Design review of the part built by this model. Coordinates are the model's own, in mm. A direction names the side the tool comes from. Give positions to 0.01 mm unless a question says otherwise; leave off trailing zeros. Write each loop counter-clockwise with the first axis right and the second up, starting at its lowest first coordinate (ties: lowest second). Pieces come first, ordered by that corner, then holes. Notation, with made-up numbers: (18.25, -28) - (43.25, -28) arc R13 ccw to (43.25, -14) - close; hole circle Ø2 at (60, -23). An arc over 180 degrees is marked (long way). Use a Markdown table: item, result. Add a question column.
```python
from build123d import *

# Parameters (mm, degrees)
ESQUISSE1_W                                       = 30
ESQUISSE1_H                                       = 30
BOSS_EXTRU_1_DEPTH                                = 38
ESQUISSE2_W                                       = 17.8
ESQUISSE2_H                                       = 4.4
ESQUISSE2_W_2                                     = 4.3
ESQUISSE2_H_2                                     = 17.8
ENL_V_MAT_EXTRU_1_DEPTH                           = 26
ESQUISSE3_W                                       = 26
ESQUISSE3_H                                       = 4.3
ENL_V_MAT_EXTRU_3_DEPTH                           = 31
ESQUISSE4_W                                       = 30
ESQUISSE4_H                                       = 3.85
BOSS_EXTRU_2_DEPTH                                = 12
FRAISAGE_POUR_VIS_T_TE_FRAIS_E_BOMB_E_D           = 5.09999996
FRAISAGE_POUR_VIS_T_TE_FRAIS_E_BOMB_E_CSINK_D     = 10.500000082
FRAISAGE_POUR_VIS_T_TE_FRAIS_E_BOMB_E_CSINK_ANGLE = 90


with BuildPart() as part:
    # Esquisse1 → Boss.-Extru.1 (new body)
    with BuildSketch(Plane(origin=(0, 0, 0), x_dir=(1, 0, 0), z_dir=(0, 1, 0))):
        with Locations((-20.886738322, -1.468531469)):
            Rectangle(ESQUISSE1_W, ESQUISSE1_H)
    extrude(amount=BOSS_EXTRU_1_DEPTH)

    # Esquisse2 → Enlèv. mat.-Extru.1 (cut)
    with BuildSketch(Plane.XZ):
        with Locations((-14.786738322, -7.431468531)):
            Rectangle(ESQUISSE2_W, ESQUISSE2_H)
        with Locations((-29.786738322, 7.568531469)):
            Rectangle(ESQUISSE2_W_2, ESQUISSE2_H_2)
        with Locations((-14.786738322, 7.568531469)):
            Rectangle(ESQUISSE2_W, ESQUISSE2_H_2)
    extrude(amount=-ENL_V_MAT_EXTRU_1_DEPTH, mode=Mode.SUBTRACT)

    # Esquisse3 → Enlèv. mat.-Extru.3 (cut, through all)
    with BuildSketch(Plane.XY.offset(16.468531469)):
        with Locations((-18.886738322, 32)):
            Rectangle(ESQUISSE3_W, ESQUISSE3_H)
    extrude(amount=-ENL_V_MAT_EXTRU_3_DEPTH, mode=Mode.SUBTRACT)

    # Esquisse4 → Boss.-Extru.2 (add)
    with BuildSketch(Plane(origin=(0, 0, -13.531468531), x_dir=(-1, 0, 0), z_dir=(0, 0, -1))):
        with Locations((20.886738322, 36.075)):
            Rectangle(ESQUISSE4_W, ESQUISSE4_H)
    extrude(amount=BOSS_EXTRU_2_DEPTH)

    # Fraisage pour vis à tête fraisée bombée #51 (through all)
    with Locations(Plane(origin=(-20.886738322, 38, -19.531468531), x_dir=(0, 0, 1), z_dir=(0, 1, 0))):
        with Locations((0, 0)):
            CounterSinkHole(FRAISAGE_POUR_VIS_T_TE_FRAIS_E_BOMB_E_D / 2, FRAISAGE_POUR_VIS_T_TE_FRAIS_E_BOMB_E_CSINK_D / 2, counter_sink_angle=FRAISAGE_POUR_VIS_T_TE_FRAIS_E_BOMB_E_CSINK_ANGLE)


solid = part.part
```
(1) Add section A-A (x = -8). State the section outline as (y, z) points, and give its area (3 significant figures).
(2) Add section C-C (y = 18). State the section outline as (x, z) points.
(3) Add section D-D (z = -11). State the section outline as (x, y) points.
(4) Mouldability with a two-part tool opening along Z and no side actions: class faces 1 (the face through (-21, 36, -25.531)), 2 (the face through (-35.887, 19, 0)), 3 (the face through (-15, 13, -5.231)), 4 (the face through (-23.687, 13, -7)) as +Z half, -Z half, draft (parallel to the pull), parting line (faces both ways), or undercut.
(5) Tool access review of faces 5 (the face through (-19, 29.85, 2)), 6 (the face through (-21, 17, -13.531)), 7 (the face through (-30, 26, 8)): name each direction out of +Z, -Z, +X, -X, +Y, -Y from which nothing blocks a thin tool from reaching the whole face with its end or side.
(6) Insertion check: pin 1 (9 mm diameter, centred on x = -12.5, z = 9, fed in from -Y); pin 2 (6.5 mm diameter, centred on x = -20.89, z = -19.53, fed in from -Y); pin 3 (14 mm diameter, centred on y = 7.5, z = 10.5, fed in from +X). Each pin has a flat end and moves straight along its axis. Give the tip position at first contact, or say it passes through.
(7) For line 1 along Y through (x, z) = (-31.75, 3.5); line 2 along X through (y, z) = (10, 10); line 3 along Z through (x, y) = (-12, 8), list the stretches that pass through material, from the lowest coordinate up.
(8) Add section B-B (z = 4). State the section outline as (x, y) points, and give its area (3 significant figures).
Answers follow:
| question | item | result |
|---|---|---|
| 1 | outline | (0, -13.53) - (29.85, -13.53) - (29.85, 16.47) - (26, 16.47) - (26, -1.33) - (0, -1.33) - (0, -5.23) - (26, -5.23) - (26, -9.63) - (0, -9.63) - close; (34.15, -25.53) - (38, -25.53) - (38, 16.47) - (34.15, 16.47) - close |
| 1 | area | 480 mm^2 |
| 2 | outline | (-35.89, -13.53) - (-5.89, -13.53) - (-5.89, -9.63) - (-23.69, -9.63) - (-23.69, -5.23) - (-5.89, -5.23) - (-5.89, -1.33) - (-23.69, -1.33) - (-23.69, 16.47) - (-27.64, 16.47) - (-27.64, -1.33) - (-31.94, -1.33) - (-31.94, 16.47) - (-35.89, 16.47) - close |
| 3 | outline | (-35.89, 0) - (-5.89, 0) - (-5.89, 29.85) - (-31.89, 29.85) - (-31.89, 34.15) - (-5.89, 34.15) - (-5.89, 38) - (-35.89, 38) - close |
| 4 | face 1 | -Z half |
| 4 | face 2 | draft |
| 4 | face 3 | undercut |
| 4 | face 4 | undercut |
| 5 | face 5 | +Z, -Z, +X |
| 5 | face 6 | -Z, +X, -X, -Y |
| 5 | face 7 | +Z, -Y |
| 6 | pin 1 | y = 26 |
| 6 | pin 2 | y = 34.15 |
| 6 | pin 3 | x = -23.69 |
| 7 | line 1 | 26 to 29.85, 34.15 to 38 |
| 7 | line 2 | -35.89 to -31.94, -27.64 to -23.69 |
| 7 | line 3 | -13.53 to -9.63, -5.23 to -1.33 |
| 8 | outline | (-35.89, 0) - (-31.94, 0) - (-31.94, 26) - (-27.64, 26) - (-27.64, 0) - (-23.69, 0) - (-23.69, 26) - (-5.89, 26) - (-5.89, 29.85) - (-31.89, 29.85) - (-31.89, 34.15) - (-5.89, 34.15) - (-5.89, 38) - (-35.89, 38) - close |
| 8 | area | 454 mm^2 |
